Answer from the drawing. Dimensions are ordinates in mm from the lowest x, y and z of the part. A direction names the side the tool comes from. Coordinates: 2 decimals unless noted, no trailing zeros. Use CSV: the item, a comma, the result in double quotes.
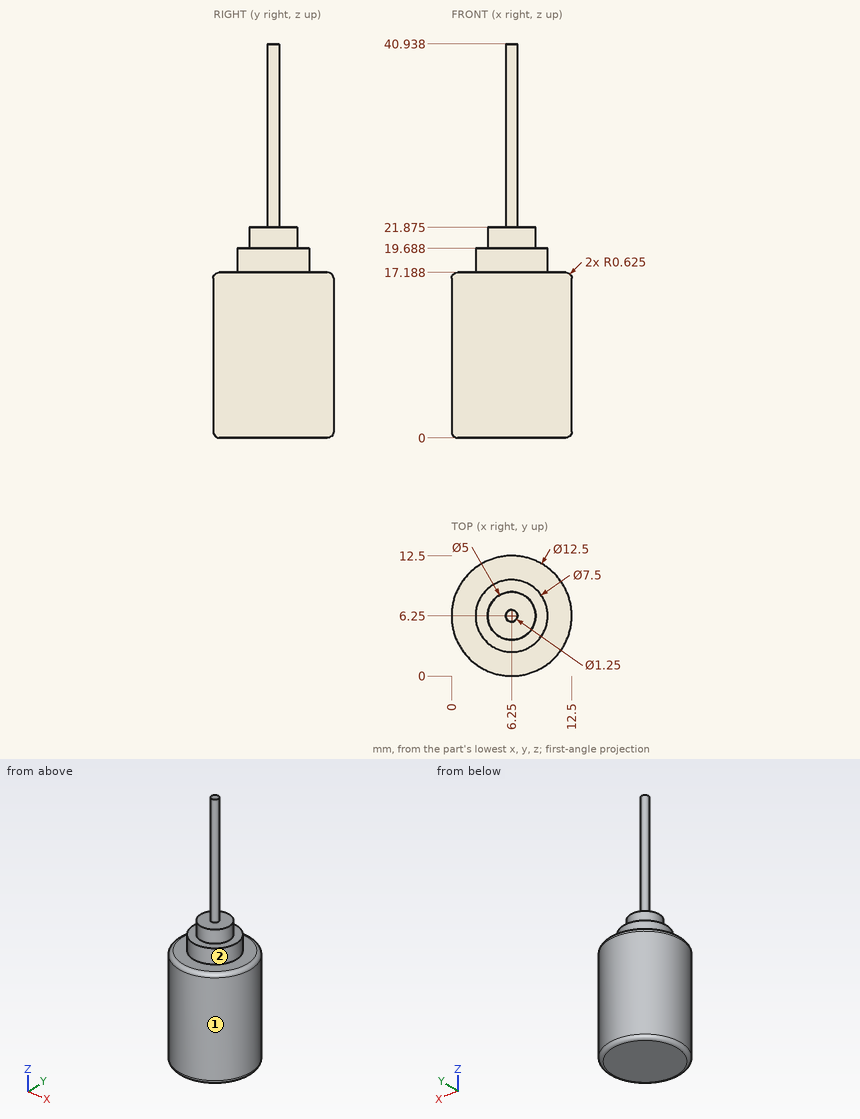
1. Find the intervals of material crossed by line 1 along X through (y, z) = (11.25, 11.5); line 2 along Z through (x, y) = (6.75, 1.5); line 3 along Z through (x, y) = (3.25, 7), in increasing order.
Solutions:
line 1,"x = 2.5 to 10"
line 2,"z = 0 to 17.19"
line 3,"z = 0 to 19.69"
2. Each of these flat-tipped pins is pushed along its axis until it touches: pin 1 Ø1.5 at (x, z) = (4, 11.5) entering from -Y; pin 2 Ø1 at (x, y) = (5.5, 9.5) entering from +Z; pin 3 Ø3 at (y, z) = (6, 7) entering from +X; pin 4 Ø3 at (x, y) = (3.5, 7) entering from +Z (1 decimal). Where does it stop, or does it pass through?
Solutions:
pin 1,"stops at y = 0.18"
pin 2,"stops at z = 19.69"
pin 3,"stops at x = 12.5"
pin 4,"stops at z = 21.9"
3. A tool of negligible diameter and unlimited length cuts with its end or side. For the marked faces 1 and 2, from which of +Z, -Z, +X, -X, +Y, -Y can it reach the whole face along a straight path? Write none if from no direction.
Solutions:
face 1,"+Z, -Z"
face 2,"+Z"
